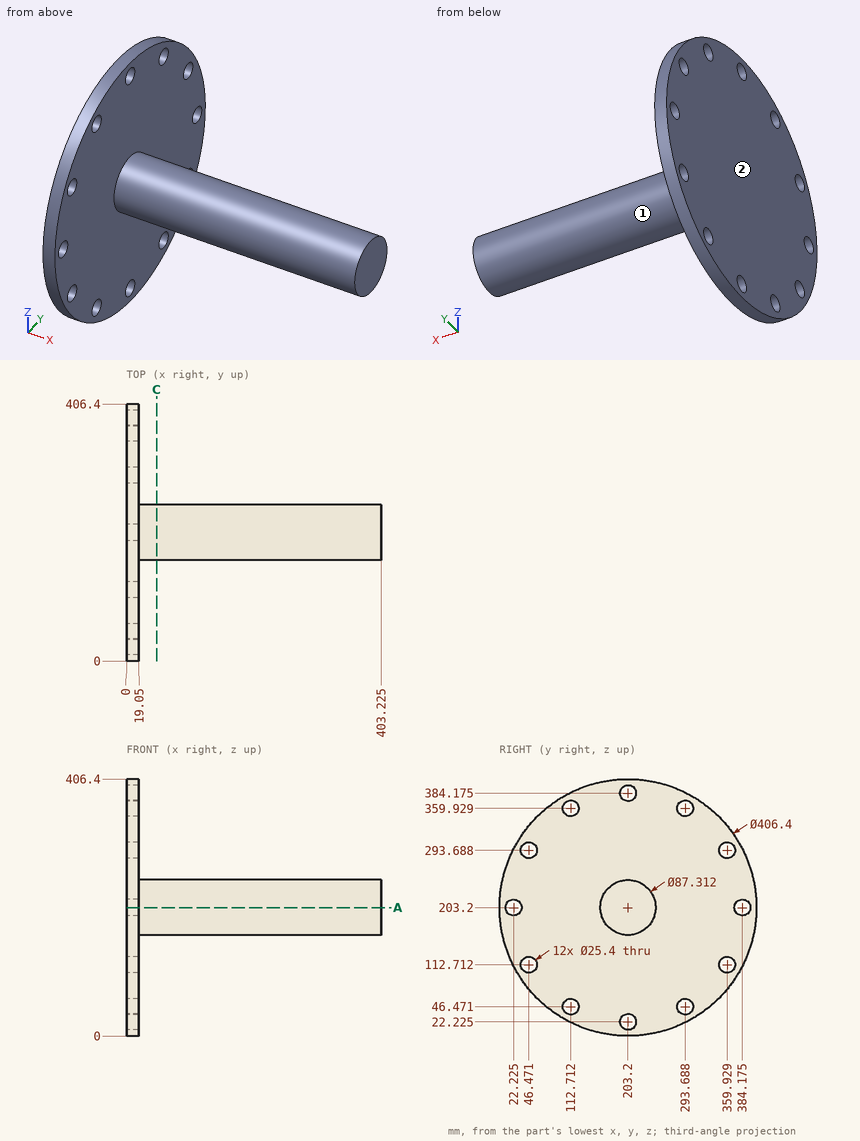
Input: dimensioned drawing with shaded views. Units: mm. Origin: part minimum x, y, z. A direction names the side the tool comes from. Give positions to 0.01 mm unless a question says otherwise; leave off trailing zeros. Loops run counter-clockwise (first coordinate to the right, second up) from the corner with the lowest first, then second, coordinate; pieces in that order, holes last. Notation, with made-up numbers: M 53,13 L 108,13 A26 ccw 108,41 Z; hole C 64,4 d3. An arc over 180 degrees is marked long. Put each result on its own line as item: value. Start each with the question number.
1) Ray query, line 1 along X through (y, z) = (54, 140.5); line 2 along Z through (x, y) = (195, 177). Return the intervals inside material, ascending.
2) Cut plane A-A (z = 203.2). Give the number of separate pieces and of enclosed holes in the cut face, then the cut area to 3 significant figures.
3) Cut plane C-C (x = 47.5). Output: boundary loops of the cut face in (y, z).
4) Access query for the marked faces 1 and 2. Directions: +Z, -Z, +X, -X, +Y, -Y. A direction counts if a zero-diameter tool reaches every point of the face in a straight line with its end or side. Return the directions, or none.
5) Contact query for flat-ended pins moving along their axis: pin 1 (12 mm diameter, centred on y = 209, z = 284.5, fed in from +X); pin 2 (12 mm diameter, centred on x = 327.5, z = 171, fed in from -Y). Output: stop coordinate, or through.
Verdict:
1. line 1: 0 to 19.05
1. line 2: 168.28 to 238.12
2. separate pieces: 3
2. enclosed holes: 0
2. area: 40,300 mm2
3. outline: C 203.2,203.2 d87.31
4. face 1: +X
4. face 2: +Z, -Z, -X, +Y, -Y
5. pin 1: x = 19.05
5. pin 2: y = 168.28
